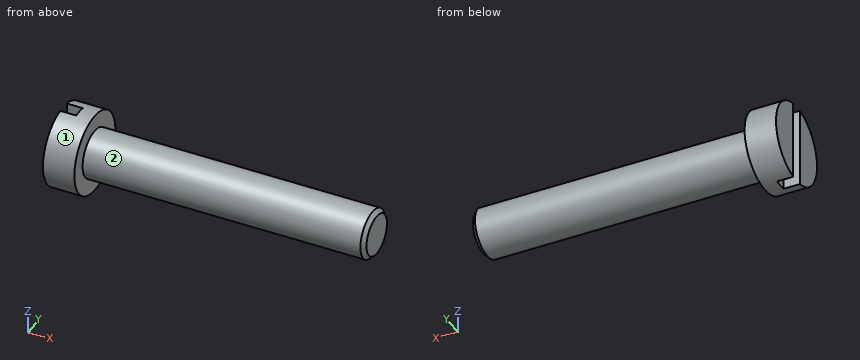
```python
from build123d import *

# Parameters (mm, degrees)
ESQUISSE2_W             = 12
ESQUISSE2_H             = 1.6
ENL_V_MAT_EXTRU_1_DEPTH = 2


with BuildPart() as part:
    # Esquisse1 → Révolution1 (revolve)
    with BuildSketch(Plane.XY, mode=Mode.PRIVATE) as r_volution1_sk:
        Polygon((0, 3), (0, 5), (-3.9, 5), (-3.9, 0), (35, 0), (35, 2.5), (34.5, 3), align=None)
    revolve(r_volution1_sk.sketch.rotate(Axis((-3.9, 0, 0), (1, 0, 0)), 90), axis=Axis((-3.9, 0, 0), (1, 0, 0)))  # turned: the seam where the file's is

    # Esquisse2 → Enlèv. mat.-Extru.1 (cut)
    with BuildSketch(Plane.ZY.offset(3.9)):
        Rectangle(ESQUISSE2_W, ESQUISSE2_H)
    extrude(amount=-ENL_V_MAT_EXTRU_1_DEPTH, mode=Mode.SUBTRACT)


solid = part.part
```
For this review, take the finished solid that the model builds, in its own axes (mm). Face numbers are marked on the shaded views. A direction names the side the tool comes from. Round coordinates to 2 decimals unless told otherwise and drop trailing zeros. Write each loop counter-clockwise with the first axis right and the second up, starting at its lowest first coordinate (ties: lowest second). Pieces come first, ordered by that corner, then holes.
1) Insertion check: pin 1 Ø1 at (x, y) = (17, 2) entering from -Z; pin 2 Ø0.6 at (x, z) = (-3, 2.5) entering from +Y; pin 3 Ø1.6 at (x, z) = (-2.5, 2.5) entering from -Y. Each pin has a flat end and moves straight along its axis. Give the tip position at first contact, or say it passes through.
Answer below:
pin 1: stops at z = -2.6
pin 2: stops at y = 4.49
pin 3: stops at y = -4.7
2) Take a section at A-A on y = 0. Give the boundary of the cut face in (x, z).
Answer below:
outline: (-1.9, -5) - (0, -5) - (0, -3) - (34.5, -3) - (35, -2.5) - (35, 2.5) - (34.5, 3) - (0, 3) - (0, 5) - (-1.9, 5) - close
3) Take a section at D-D on z = 4. Give the boundary of the cut face in (x, y), then the cut area to 3 significant figures.
Answer below:
outline: (-3.9, -3) - (0, -3) - (0, 3) - (-3.9, 3) - (-3.9, 0.8) - (-1.9, 0.8) - (-1.9, -0.8) - (-3.9, -0.8) - close
area: 20.2 mm2
4) Take a section at B-B on z = 0. Give the boundary of the cut face in (x, y).
Answer below:
outline: (-3.9, -5) - (0, -5) - (0, -3) - (34.5, -3) - (35, -2.5) - (35, 2.5) - (34.5, 3) - (0, 3) - (0, 5) - (-3.9, 5) - (-3.9, 0.8) - (-1.9, 0.8) - (-1.9, -0.8) - (-3.9, -0.8) - close
5) Machinability: for the marked faces 1 and 2, which of the approach directions +Z, -Z, +X, -X, +Y, -Y give a long, thin tool a straight path to every point of the face, cutting with its end or side? Answer none if there is none.
Answer below:
face 1: +X, -X
face 2: +X
6) For line 1 along X through (y, z) = (-3, 1); line 2 along X through (y, z) = (-0.5, 0.25); line 3 along Y through (x, z) = (-2, 0.5), list the stretches that pass through material, from the lowest coordinate up.
Answer below:
line 1: x = -3.9 to 0
line 2: x = -1.9 to 35
line 3: y = -4.97 to -0.8, 0.8 to 4.97
7) Take a section at C-C on x = 3. Give the boundary of the cut face in (y, z), then the cut area to 3 significant figures.
Answer below:
outline: circle Ø6 at (0, 0)
area: 28.3 mm2
